Work out the finished part from the listing and answer in its coordinate system (mm). A direction names the side the tool comes from. Coordinates: 2 decimals unless noted, no trailing zeros. Write each loop counter-clockwise with the first axis right and the second up, starting at its lowest first coordinate (ties: lowest second). Pieces come first, ordered by that corner, then holes. Notation, with made-up numbers: (15.25, 55.5) - (28.25, 55.5) arc R5 ccw to (28.25, 63.5) - close; hole circle Ø5 at (-4.5, 49.5). An arc over 180 degrees is marked (long way). Answer as a JSON object with one key per item and string values. Group by question number.
from build123d import *

# Parameters (mm, degrees)
SKETCH_5_W          = 23
SKETCH_5_H          = 22.5
EXTRUDE_4_DEPTH     = 12.6
SKETCH_6_W          = 32.4
SKETCH_6_H          = 2.4
EXTRUDE_5_DEPTH     = 12.6
SKETCH_7_R          = 6.3
EXTRUDE_6_DEPTH     = 4.2
SKETCH_9_R          = 2.3
EXTRUDE_8_DEPTH     = 2.5
SKETCH_10_R         = 0.9
CUT_EXTRUDE_1_DEPTH = 2.5
M2X0_4_1_D          = 1.6


with BuildPart() as part:
    # ｽｹｯﾁ5 → ﾎﾞｽ - 押し出し4 (new body)
    with BuildSketch(Plane.XY):
        Rectangle(SKETCH_5_W, SKETCH_5_H)
    extrude(amount=EXTRUDE_4_DEPTH)

    # ｽｹｯﾁ6 → ﾎﾞｽ - 押し出し5 (add)
    with BuildSketch(Plane.XY):
        with Locations((-0.05, 5.75)):
            Rectangle(SKETCH_6_W, SKETCH_6_H)
    extrude(amount=EXTRUDE_5_DEPTH)

    # ｽｹｯﾁ7 → ﾎﾞｽ - 押し出し6 (add)
    with BuildSketch(Plane(origin=(0, 11.25, 0), x_dir=(1, 0, 0), z_dir=(0, 1, 0))):
        with Locations(Location((5.2, -6.3, 0), (0, 0, 270))):
            Circle(SKETCH_7_R)
    extrude(amount=EXTRUDE_6_DEPTH)

    # ｽｹｯﾁ9 → ﾎﾞｽ - 押し出し8 (add)
    with BuildSketch(Plane(origin=(0, 15.45, 0), x_dir=(1, 0, 0), z_dir=(0, 1, 0))):
        with Locations(Location((5.2, -6.3, 0), (0, 0, 270))):
            Circle(SKETCH_9_R)
    extrude(amount=EXTRUDE_8_DEPTH)

    # ｽｹｯﾁ10 → ｶｯﾄ - 押し出し1 (cut)
    with BuildSketch(Plane(origin=(0, 15.45, 0), x_dir=(1, 0, 0), z_dir=(0, 1, 0))):
        with Locations(Location((5.2, -6.3, 0), (0, 0, 270))):
            Circle(SKETCH_10_R)
    extrude(amount=CUT_EXTRUDE_1_DEPTH, mode=Mode.SUBTRACT)

    # M2x0.4 ねじ穴1 (through all)
    with Locations(Plane(origin=(0, 6.95, 0), x_dir=(1, 0, 0), z_dir=(0, 1, 0))):
        with Locations((-13.9, -6.3), (13.9, -6.3)):
            Hole(M2X0_4_1_D / 2)


solid = part.part
Q1. A tool of negligible diameter and unlimited length cuts with its end or side. For faces 1 (the face through (12.8, 4.55, 6.2)), 2 (the face through (10, 11.25, 1)), 3 (the face through (2, 15.45, 6)), 4 (the face through (-11.5, 9, 6)), from which of +Z, -Z, +X, -X, +Y, -Y can it reach the whole face along a straight path? Write none if from no direction.
Q2. Section A-A on x = -13.9 is taken. Determine the outline of the cut face in (y, z).
Q3. Flat-ended cylindrical pins translate along their axes: pin 1 Ø6.5 at (x, z) = (-7.5, 9) entering from +Y; pin 2 Ø0.9 at (x, z) = (5.5, 6.5) entering from +Y; pin 3 Ø1.4 at (x, z) = (14, 4) entering from +Y. Find the tip coordinate at first contact, or state that the pin passes through.
Q4. For a pull along Z with two mould halves and no side action, classify faces 5 (the face through (0, 0, 0)), 6 (the face through (5.47, 16.68, 7.16)), 7 (the face through (10, 11.25, 11)), 8 (the face through (5, 15.45, 6)) as +Z half, -Z half, draft (parallel to the pull), parting line (faces both ways), or undercut.
Q5. Consider L1, parallel to X at y = 5.5, z = 6.3; L2, parallel to Z at x = -13.9, y = 6.3; L3, parallel to X at y = 17.3, z = 6.3. Determine where each line is inside the solid, lowest interval first. Write a range as from..to.
Q6. Section B-B on z = 4.5 is taken. Determine the outline of the cut face in (x, y), plus the area to 3 significant figures.
Q7. Section C-C on y = 13.5 is taken. Determine the outline of the cut face in (x, z).
Q8. Section D-D on x = -1.5 is taken. Determine the outline of the cut face in (y, z).
Numbers:
{
 "1": {"face 1": "+Z, -Z, +X, -Y", "face 2": "-Z, +X, +Y", "face 3": "+Y", "face 4": "+Z, -Z, -X, +Y"},
 "2": {"outline": "(4.55, 0) - (6.95, 0) - (6.95, 5.5) - (4.55, 5.5) - close; (4.55, 7.1) - (6.95, 7.1) - (6.95, 12.6) - (4.55, 12.6) - close"},
 "3": {"pin 1": "stops at y = 11.25", "pin 2": "stops at y = 15.45", "pin 3": "stops at y = 6.95"},
 "4": {"face 5": "-Z half", "face 6": "undercut", "face 7": "draft", "face 8": "undercut"},
 "5": {"L1": "x = -16.25..-14.7, -13.1..13.1, 14.7..16.15", "L2": "z = 0..5.5, 7.1..12.6", "L3": "x = 2.9..4.3, 6.1..7.5"},
 "6": {"outline": "(-16.25, 4.55) - (-11.5, 4.55) - (-11.5, -11.25) - (11.5, -11.25) - (11.5, 4.55) - (16.15, 4.55) - (16.15, 6.95) - (11.5, 6.95) - (11.5, 11.25) - (11.24, 11.25) - (11.24, 15.45) - (6.63, 15.45) - (6.63, 17.95) - (3.77, 17.95) - (3.77, 15.45) - (-0.84, 15.45) - (-0.84, 11.25) - (-11.5, 11.25) - (-11.5, 6.95) - (-16.25, 6.95) - close", "area": "598 mm²"},
 "7": {"outline": "circle Ø12.6 at (5.2, 6.3)"},
 "8": {"outline": "(-11.25, 0) - (11.25, 0) - (11.25, 12.6) - (-11.25, 12.6) - close"}
}
